Autodesk Inventor part; units mm, degrees
ref_plane "Plan de construction1" through (0, 0, 0) normal (0.7071068, -0.7071068, 0) x (0, 0, -1)
ref_plane "XY Plane" through (0, 0, 0) normal (0, 0, 1) x (1, 0, 0)
sketch "Esquisse1" plane through (0, 0, 0) normal (0, 0, 1) x (1, 0, 0)
  circle A0 centre (0, 0) radius 5.5
  dimension "d0" = 11
extrude "Extrusion1" add sketch "Esquisse1" along normal blind 15
ref_plane "Plan de construction1" through (0, 0, 0) normal (0.7071068, -0.7071068, 0) x (0, 0, -1)
sketch "Esquisse3" plane through (0, 0, 0) normal (0.7071068, -0.7071068, 0) x (0, 0, -1)
  circle A0 centre (-9, -7) radius 3
  line L0 (-15, 5.5) -> (-15, -5.5)
  line L1 (0, -5.5) -> (0, 5.5)
  point P0 (0, 0)
  dimension "d3" = 6
  dimension "d4" = 7
  dimension "d5" = 15
  dimension "d6" = 9
extrude "Extrusion2" add sketch "Esquisse3" along normal mid plane 11
sketch "Esquisse4" plane through (-8.8388, -1.0607, 9) normal (-0.7071068, 0.7071068, 0) x (-0.7071068, -0.7071068, 0)
  circle A0 centre (0, 0) radius 2
  point P0 (-7, -9)
  dimension "d9" = 4
extrude "Extrusion3" cut sketch "Esquisse4" against normal through all
sketch "Esquisse5" plane through (0, 0, 15) normal (0, 0, 1) x (1, 0, 0)
  line L0 (-6.9282, 0) -> (-3.4641, 6)
  line L1 (-3.4641, 6) -> (3.4641, 6)
  line L2 (3.4641, 6) -> (6.9282, 0)
  line L3 (6.9282, 0) -> (3.4641, -6)
  line L4 (3.4641, -6) -> (-3.4641, -6)
  line L5 (-3.4641, -6) -> (-6.9282, 0)
  point P0 (0, 0)
  point P1 (0, 0)
  dimension "d12" = 12
extrude "Extrusion4" add sketch "Esquisse5" along normal blind 6
sketch "Esquisse6" plane through (0, 0, 21) normal (0, 0, 1) x (1, 0, 0)
  circle A0 centre (0, 0) radius 2
  dimension "d15" = 4
extrude "Extrusion5" add sketch "Esquisse6" along normal blind 7
thread "Filetage1"
fillet "Congé1" radius 0.5 1 edges at (-2, 0, 28)
sketch "Esquisse8" plane through (0, 0, 0) normal (0.7071068, -0.7071068, 0) x (0, 0, -1)
  line L0 (0, -5.5) -> (0, 5.5)
  line L1 (0, 3.5) -> (-9, 3.5)
  line L2 (-9, 3.5) -> (-9, 17.5)
  line L3 (-9, 17.5) -> (0, 17.5)
  line L4 (0, 17.5) -> (0, 3.5)
  point P0 (0, 0)
  dimension "d21" = 3.5
  dimension "d22" = 14
  dimension "d23" = 9
extrude "Extrusion6" add sketch "Esquisse8" along normal mid plane 3
sketch "Esquisse9" plane through (-1.0607, 1.0607, 0) normal (-0.7071068, 0.7071068, 0) x (-0.7071068, -0.7071068, 0)
  line L0 (-5.2915, 9) -> (-5.2915, 0)
  line L1 (-5.2915, 9) -> (-17.5, 6)
  line L2 (-17.5, 9) -> (-17.5, 0)
  line L3 (-5.2915, 9) -> (-17.5, 9)
  line L4 (-17.5, 9) -> (-5.2915, 9)
  point P0 (0, 0)
  dimension "d26" = 6
extrude "Extrusion7" cut sketch "Esquisse9" against normal blind 3
sketch "Esquisse10" plane through (-1.0607, 1.0607, 0) normal (-0.7071068, 0.7071068, 0) x (-0.7071068, -0.7071068, 0)
  circle A0 centre (-14.5, 3) radius 1.5
  line L0 (-17.5, 0) -> (-5.2915, 0)
  line L1 (-17.5, 6) -> (-17.5, 0)
  point P0 (0, 0)
  dimension "d29" = 3
  dimension "d30" = 3
  dimension "d31" = 3
extrude "Extrusion8" cut sketch "Esquisse10" against normal through all
fillet "Congé2" radius 3 2 edges at (12.3744, 12.3744, 0) (12.3744, 12.3744, 6)
fillet "Congé3" radius 1 2 edges at (2.681, 4.8023, 4.5) (4.8023, 2.681, 4.5)
properties part number "Fusée" material "Acier inoxydable"
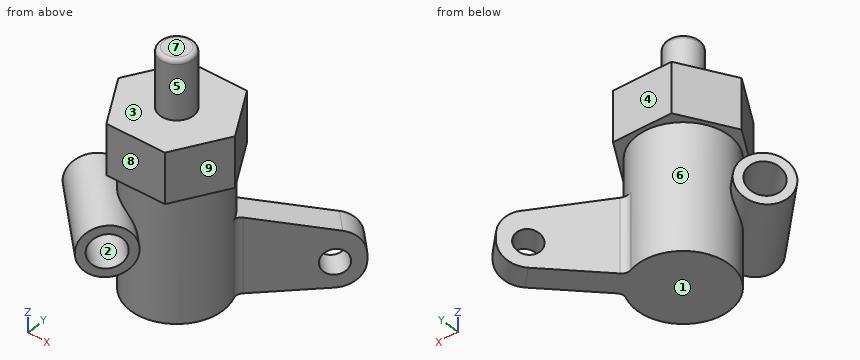
Model file for the job. Use its own axes, mm. Face numbers are marked on the shaded views. A direction names the side the tool comes from. Coordinates: 2 decimals unless noted, no trailing zeros. Loops run counter-clockwise (first coordinate to the right, second up) from the corner with the lowest first, then second, coordinate; pieces in that order, holes last. Notation, with made-up numbers: M 72,65 L 118,65 A18 cw 118,97 Z; hole C 34.5,66 d11. An arc over 180 degrees is marked long. Use CSV: the item, a comma, the result in double quotes. Start each with the question number.
1. Band-saw the part on A-A, the plane z = 19. List the corners of the cut face in (x, y).
2. Band-saw the part on B-B, the plane z = 22.25. List the corners of the cut face in (x, y), then the cut area to 3 significant figures.
3. Probe probe 1 along Z at (x, y) = (2.5, -3.5); probe 2 along Z at (x, y) = (-2.25, 5.25); probe 3 along Y at (x, z) = (-7.5, 10). List the from-to ranges inside material, lowest first. Write a range as [from, to].
4. Flat gauge pins, fed straight in: pin 1 (13 mm diameter, centred on x = 0.5, y = 2, fed in from +Z); pin 2 (4 mm diameter, centred on x = -8, y = 1.5, fed in from +Z); pin 3 (6 mm diameter, centred on x = -6, z = 13.5, fed in from -Y); pin 4 (12 mm diameter, centred on y = -1, z = 10, fed in from +X). Where does each tip first touch, or does it go through?
5. Tool access for the marked faces 5, 6, 7, 8 and 9: list every direction of +Z, -Z, +X, -X, +Y, -Y with a clear straight run to the whole face (end or side of a thin tool).
6. Two-plate mould, pull along Z, no slides. Class the marked faces 1, 2, 3 and 4: pulls with the +Z half, pulls with the -Z half, needs draft (parallel to the pull), parting line crosses it, or undercut.
Entries:
1,outline,"M -6.93,0 L -3.46,-6 L 3.46,-6 L 6.93,0 L 3.46,6 L -3.46,6 Z"
2,outline,"C 0,0 d4"
2,area,"12.6 mm2"
3,probe 1,"z = [0, 21]"
3,probe 2,"z = [15, 21]"
3,probe 3,"y = [-6.4, -4.85], [0.05, 0.28]"
4,pin 1,"stops at z = 28"
4,pin 2,"stops at z = 21"
4,pin 3,"stops at y = -8.73"
4,pin 4,"stops at x = 6.93"
5,face 5,"+Z"
5,face 6,"none"
5,face 7,"+Z, +X, -X, +Y, -Y"
5,face 8,"+Z, +X, -X, -Y"
5,face 9,"+Z, -Z, +X, -Y"
6,face 1,"pulls with the -Z half"
6,face 2,"undercut"
6,face 3,"pulls with the +Z half"
6,face 4,"needs draft"
